Can you work these out from the model? Positions are in its coordinate system, mm. Face numbers are marked on the shaded views. A direction names the side the tool comes from. Round coordinates to 2 decimals unless told otherwise and drop trailing zeros. Write each loop counter-clockwise with the first axis right and the second up, starting at its lowest first coordinate (ties: lowest second). Pieces come first, ordered by that corner, then holes. Notation, with made-up numbers: (54.25, 10) -> (86.25, 10) arc R8 cw to (86.25, 23) -> close; hole circle Ø9 at (-2, 7). An arc over 180 degrees is marked (long way). Write item = value, one per line. Start each with the question number.
1) Imagine slicing it at D-D, the plane z = 4.25. Please give me the cut outline in (x, y).
2) Imagine slicing it at C-C, the plane x = 18. Please give me the cut outline in (y, z).
3) Imagine slicing it at B-B, the plane y = 13.15. Please give me the cut outline in (x, z), then the cut area to 3 significant figures.
4) If I drill on line 1 (Y direction, x = 4.25, z = 3.5); line 2 (X direction, y = 16.25, z = 1.5); line 3 (Y direction, x = 24.75, z = 1.5), over which ranges is the centre line in solid material (lowest first)?
5) Thinking about a two-plate mould opening in X: for the marked faces 1, 2 and 3, which applies, +X half, -X half, draft (parallel to the pull), parting line (faces both ways), or undercut?
6) For the marked faces 4 and 5, which set-ups out of +Z, -Z, +X, -X, +Y, -Y let a thin tool reach every point of the face, with its end or its side?
7) I'm going to push flat-ended pins straight in: pin 1 (2 mm diameter, centred on x = 24.5, y = 11, fed in from +Z); pin 2 (6 mm diameter, centred on x = 19, y = 10.5, fed in from +Z); pin 3 (3 mm diameter, centred on x = 11, z = 3, fed in from -Y). Where does each tip first touch, or does it pass through?
8) Imagine slicing it at A-A, the plane z = 2. Please give me the cut outline in (x, y), then the cut area to 3 significant figures.
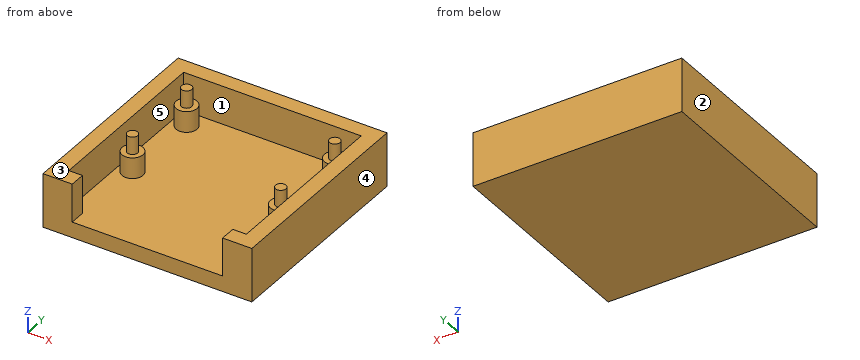
from build123d import *

# Parameters (mm, degrees)
F1_DEPTH = 5.5
F0_W     = 21.6
F0_H     = 2.25
F2_DEPTH = 2.25
F3_R     = 1.5
F3_R_2   = 0.75
F4_DEPTH = 3
F5_DEPTH = 5.5


with BuildPart() as f1:
    # F0 (on Top) → F1 (new body)
    with BuildSketch(Plane.XY):
        Polygon((0, 30), (0, 0), (4.2, 0), (4.2, 2.25), (2.25, 2.25), (2.25, 27.75), (27.75, 27.75), (27.75, 2.25), (25.8, 2.25), (25.8, 0), (30, 0), (30, 30), align=None)
    extrude(amount=F1_DEPTH)

    # F0 (on Top) → F2 (join)
    with BuildSketch(Plane.XY):
        Polygon((2.25, 2.25), (4.2, 2.25), (25.8, 2.25), (27.75, 2.25), (27.75, 27.75), (2.25, 27.75), align=None)
        Polygon((0, 30), (0, 0), (4.2, 0), (4.2, 2.25), (2.25, 2.25), (2.25, 27.75), (27.75, 27.75), (27.75, 2.25), (25.8, 2.25), (25.8, 0), (30, 0), (30, 30), align=None)
        with Locations((15, 1.125)):
            Rectangle(F0_W, F0_H)
    extrude(amount=-F2_DEPTH)

    # F3 (on face) → F4 (join)
    with BuildSketch(Plane.XY):
        with Locations((25.65, 25.15)):
            Circle(F3_R)
        with Locations((25.65, 25.15)):
            Circle(F3_R_2, mode=Mode.SUBTRACT)
        with Locations((25.65, 13.15)):
            Circle(F3_R)
        with Locations((25.65, 13.15)):
            Circle(F3_R_2, mode=Mode.SUBTRACT)
        with Locations((4.35, 25.15)):
            Circle(F3_R)
        with Locations((4.35, 25.15)):
            Circle(F3_R_2, mode=Mode.SUBTRACT)
        with Locations((4.35, 13.15)):
            Circle(F3_R)
        with Locations((4.35, 13.15)):
            Circle(F3_R_2, mode=Mode.SUBTRACT)
    extrude(amount=F4_DEPTH)

    # F3 (on face) → F5 (join)
    with BuildSketch(Plane.XY):
        with Locations((4.35, 25.15)):
            Circle(F3_R_2)
        with Locations((25.65, 25.15)):
            Circle(F3_R_2)
        with Locations((25.65, 13.15)):
            Circle(F3_R_2)
        with Locations((4.35, 13.15)):
            Circle(F3_R_2)
    extrude(amount=F5_DEPTH)


solid = f1.part
Reported:
q1.outline = (0, 0) -> (4.2, 0) -> (4.2, 2.25) -> (2.25, 2.25) -> (2.25, 27.75) -> (27.75, 27.75) -> (27.75, 2.25) -> (25.8, 2.25) -> (25.8, 0) -> (30, 0) -> (30, 30) -> (0, 30) -> close; circle Ø1.5 at (4.35, 13.15); circle Ø1.5 at (4.35, 25.15); circle Ø1.5 at (25.65, 13.15); circle Ø1.5 at (25.65, 25.15)
q2.outline = (0, -2.25) -> (30, -2.25) -> (30, 5.5) -> (27.75, 5.5) -> (27.75, 0) -> (0, 0) -> close
q3.outline = (0, -2.25) -> (30, -2.25) -> (30, 5.5) -> (27.75, 5.5) -> (27.75, 0) -> (27.15, 0) -> (27.15, 3) -> (26.4, 3) -> (26.4, 5.5) -> (24.9, 5.5) -> (24.9, 3) -> (24.15, 3) -> (24.15, 0) -> (5.85, 0) -> (5.85, 3) -> (5.1, 3) -> (5.1, 5.5) -> (3.6, 5.5) -> (3.6, 3) -> (2.85, 3) -> (2.85, 0) -> (2.25, 0) -> (2.25, 5.5) -> (0, 5.5) -> close
q3.area = 118 mm²
q4.line_1 = 12.41 to 13.89, 24.41 to 25.89, 27.75 to 30
q4.line_2 = 0 to 2.25, 27.75 to 30
q4.line_3 = 11.95 to 14.35, 23.95 to 26.35, 27.75 to 30
q5.face_1 = undercut
q5.face_2 = -X half
q5.face_3 = draft
q6.face_4 = +Z, -Z, +X, +Y, -Y
q6.face_5 = +Z
q7.pin_1 = 3
q7.pin_2 = 0
q7.pin_3 = 27.75
q8.outline = (0, 0) -> (4.2, 0) -> (4.2, 2.25) -> (2.25, 2.25) -> (2.25, 27.75) -> (27.75, 27.75) -> (27.75, 2.25) -> (25.8, 2.25) -> (25.8, 0) -> (30, 0) -> (30, 30) -> (0, 30) -> close; circle Ø3 at (4.35, 13.15); circle Ø3 at (4.35, 25.15); circle Ø3 at (25.65, 13.15); circle Ø3 at (25.65, 25.15)
q8.area = 229 mm²
